Here's the drawing with two shaded views (mm, measured from the low corner). I have some questions. Give positions to 0.01 mm unless a question says otherwise; leave off trailing zeros. Order: outer loops, then holes, each group sorted by start corner. A loop starts at its lowest first (then second) coordinate and runs counter-clockwise, first axis right, second up. Notation, with made-up numbers: (14, 21.25) - (41, 21.25) arc R16 ccw to (41, 36.25) - close; hole circle Ø11 at (-32, -19.75). An arc over 180 degrees is marked (long way). Use one line per item in the form item = value. Start each with the question number.
1) Please list where these lines run through material, in increasing order: probe 1 along Y at (x, z) = (86, 2.45); probe 2 along Y at (x, z) = (126, 1.9); probe 3 along Y at (x, z) = (107.5, 1.65).
2) Suppose I cut it at C-C, the plane z = 1.65. State how many separate pieces and enclosed holes the cut face has, and give its area (3 significant figures).
3) Suppose I cut it at A-A, the plane y = 28. Write out the boundary of the cut face in (x, z).
4) Suppose I cut it at B-B, the plane x = 86. Write out the boundary of the cut face in (y, z), and give its area (3 significant figures).
5) For pin 1 (2 mm diameter, centred on y = 35, z = 2, fed in from -X), with a flat end and sliding along its axis, tell me the tip position at first contact or that it passes through.
6) Suppose I cut it at D-D, the plane x = 106. Write out the boundary of the cut face in (y, z), and give its area (3 significant figures).
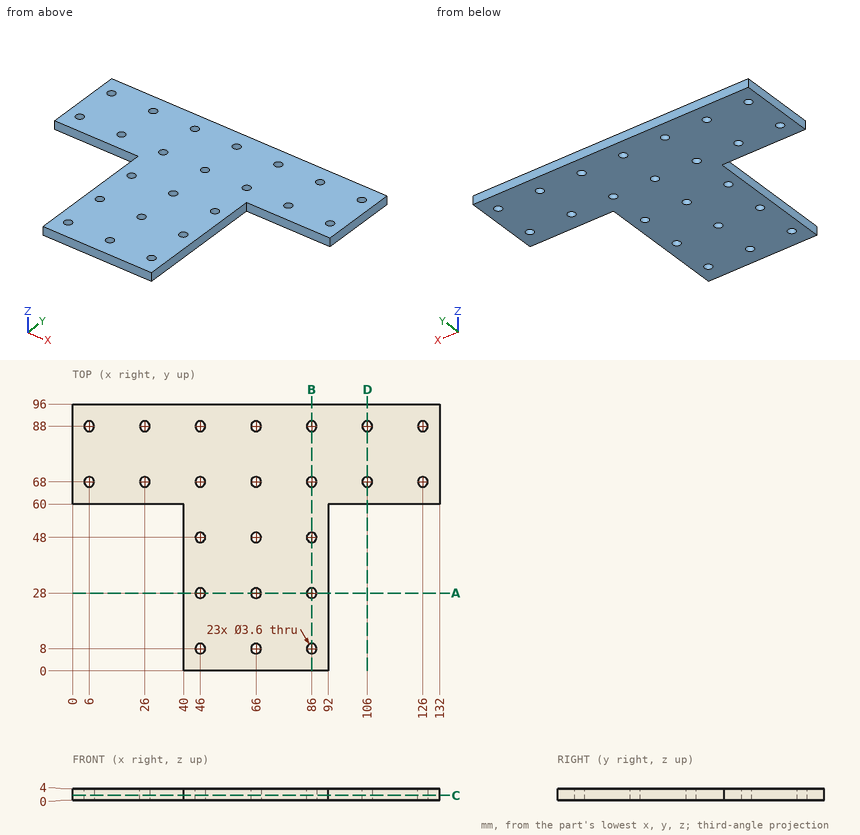
Result sheet:
q1.probe_1 = 0 to 6.2, 9.8 to 26.2, 29.8 to 46.2, 49.8 to 66.2, 69.8 to 86.2, 89.8 to 96
q1.probe_2 = 60 to 66.2, 69.8 to 86.2, 89.8 to 96
q1.probe_3 = 60 to 67.01, 68.99 to 87.01, 88.99 to 96
q2.separate_pieces = 1
q2.enclosed_holes = 23
q2.area = 7,640 mm²
q3.outline = (40, 0) - (44.2, 0) - (44.2, 4) - (40, 4) - close; (47.8, 0) - (64.2, 0) - (64.2, 4) - (47.8, 4) - close; (67.8, 0) - (84.2, 0) - (84.2, 4) - (67.8, 4) - close; (87.8, 0) - (92, 0) - (92, 4) - (87.8, 4) - close
q4.outline = (0, 0) - (6.2, 0) - (6.2, 4) - (0, 4) - close; (9.8, 0) - (26.2, 0) - (26.2, 4) - (9.8, 4) - close; (29.8, 0) - (46.2, 0) - (46.2, 4) - (29.8, 4) - close; (49.8, 0) - (66.2, 0) - (66.2, 4) - (49.8, 4) - close; (69.8, 0) - (86.2, 0) - (86.2, 4) - (69.8, 4) - close; (89.8, 0) - (96, 0) - (96, 4) - (89.8, 4) - close
q4.area = 312 mm²
q5.pin_1 = 40
q6.outline = (60, 0) - (66.2, 0) - (66.2, 4) - (60, 4) - close; (69.8, 0) - (86.2, 0) - (86.2, 4) - (69.8, 4) - close; (89.8, 0) - (96, 0) - (96, 4) - (89.8, 4) - close
q6.area = 115 mm²
